Part print with two shaded views. Sizes in mm from the minimum x, y, z corner. Give positions to 0.01 mm unless a question says otherwise; leave off trailing zeros. Write each loop counter-clockwise with the first axis right and the second up, starting at its lowest first coordinate (ties: lowest second). Pieces come first, ordered by that corner, then holes.
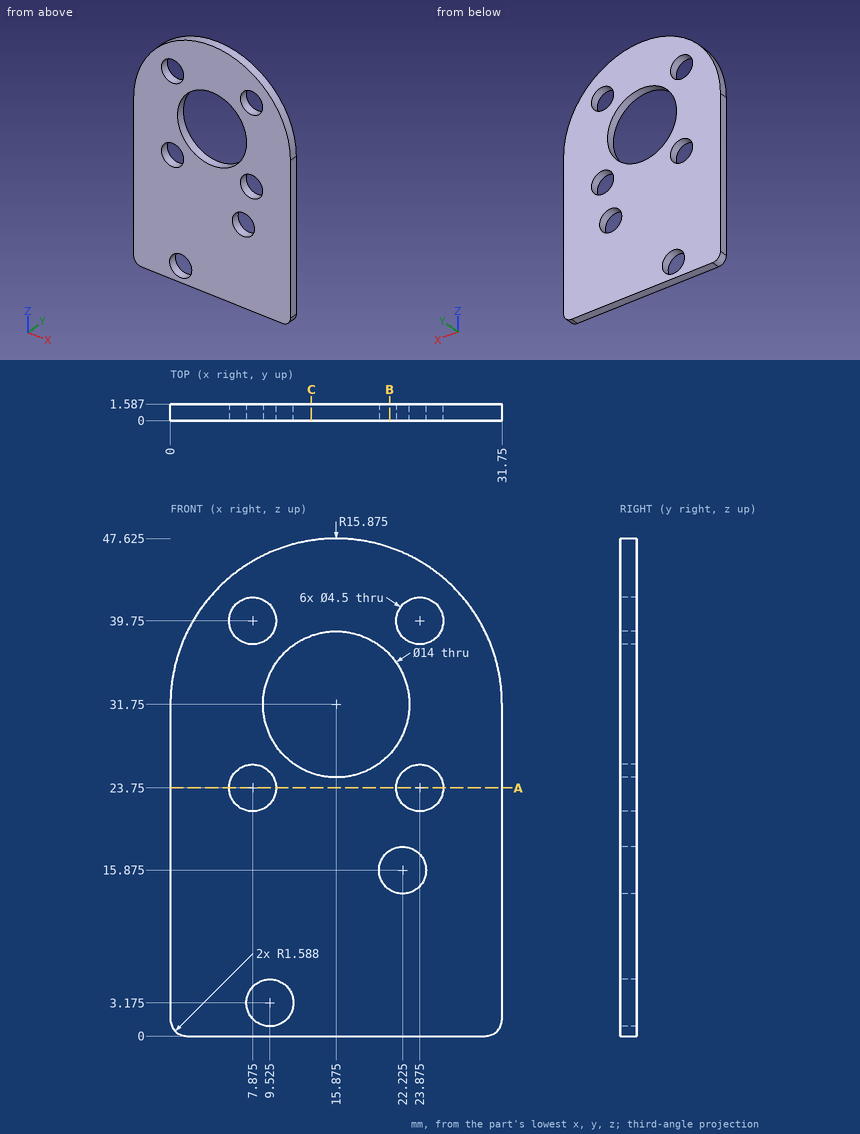
1) Saw through at A-A, the plane z = 23.75. Count the separate pieces of the cut face and the enclosed holes in it.
Answers follow:
separate pieces: 3
enclosed holes: 0
2) Pin check, flat tip, straight feed: pin 1 Ø2.5 at (x, z) = (7.875, 23.75) entering from -Y. Stop position of the tip, or through.
Answers follow:
pin 1: passes through
3) Saw through at B-B, the plane x = 21. Write the cut outline in (y, z) (1 decimal).
Answers follow:
outline: (0, 0) - (1.6, 0) - (1.6, 14) - (0, 14) - close; (0, 17.8) - (1.6, 17.8) - (1.6, 27) - (0, 27) - close; (0, 36.5) - (1.6, 36.5) - (1.6, 46.8) - (0, 46.8) - close
4) Wall check: L1, parallel to Z at x = 23.5, y = 1.15 (1 decimal); L2, parallel to Z at x = 7, y = 0.2 (1 decimal); L3, parallel to X at y = 1.05, z = 16. Give the ranges that are in metal, low to high.
Answers follow:
L1: z = 0 to 14, 17.7 to 21.5, 26 to 37.5, 42 to 45.7
L2: z = 0 to 21.7, 25.8 to 37.7, 41.8 to 44.9
L3: x = 0 to 19.98, 24.47 to 31.75
5) Saw through at C-C, the plane x = 13.5. Write the cut outline in (y, z) (1 decimal).
Answers follow:
outline: (0, 0) - (1.6, 0) - (1.6, 25.2) - (0, 25.2) - close; (0, 38.3) - (1.6, 38.3) - (1.6, 47.4) - (0, 47.4) - close
